Can you work these out from the model? Positions are in its coordinate system, mm. Face numbers are marked on the shaded views. Coordinates: 2 decimals unless noted, no trailing zeros. Order: outer loops, then holes, each group sorted by start corner. A loop starts at its lowest first (then second) coordinate and runs counter-clockwise, first axis right, second up. Notation, with made-up numbers: M -19,25.5 L 0,25.5 A21 ccw 0,45.5 Z; hole C 4.5,15.5 d3. An arc over 180 degrees is marked long. Answer as CSV lines item,"result". Start each with the question number.
1. If we section it at D-D (x = 0): List the corners of the cut face in (y, z) for me.
2. If we section it at A-A (y = 2): List the corners of the cut face in (x, z) for me, plus the area to 3 significant figures.
3. If we section it at C-C (z = 5): List the corners of the cut face in (x, y) for me, plus the area to 3 significant figures.
4. If we mould it in two halves opening along X, with no side actions, what happens to the marked faces 1, 2, 3 and 4? For each: released by +X, released by -X, zero draft, split by the parting line, or undercut.
5. If we section it at B-B (x = 2): List the corners of the cut face in (y, z) for me.
6. I need wall thicknesses on line 1 along Z through (x, y) = (0, 1); line 2 along X through (y, z) = (1, 3.75); line 3 along Z through (x, y) = (1, 4). Which ranges of each line are inside material? Lowest first, please. Write a range as from..to.
```python
from build123d import *

# Parameters (mm, degrees)
F0_W     = 10
F0_H     = 10
F1_DEPTH = 10
F2_R     = 2.5
F3_DEPTH = 10.1
F4_R     = 1


with BuildPart() as f1:
    # F0 (on Top) → F1 (new body)
    with BuildSketch(Plane.XY):
        Rectangle(F0_W, F0_H)
    extrude(amount=F1_DEPTH)

    # F2 (on face) → F3 (cut)
    with BuildSketch(Plane.XZ.offset(5)):
        with Locations((0, 5)):
            Circle(F2_R)
    extrude(amount=-F3_DEPTH, mode=Mode.SUBTRACT)

    # F4
    f4_edges = [f1.edges().sort_by_distance(p)[0] for p in [
        (5, 0, 10),
        (0, 5, 10),
        (-5, 0, 10),
        (0, -5, 10),
        (5, 0, 0),
        (0, 5, 0),
        (-5, 0, 0),
        (0, -5, 0),
    ]]
    fillet(f4_edges, radius=F4_R)


solid = f1.part
```
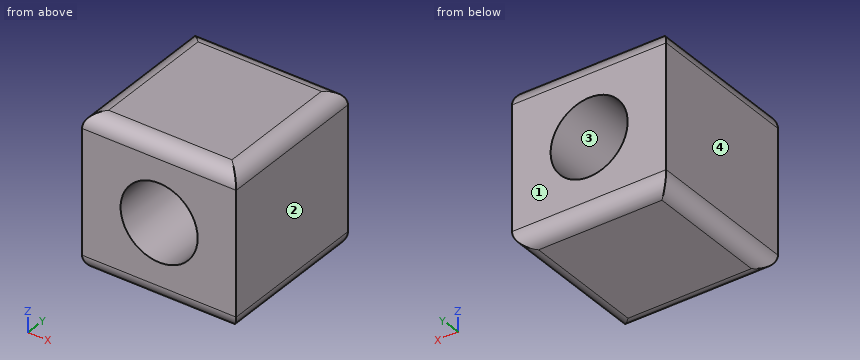
Solved:
1,outline,"M -5,1 A1 ccw -4,0 L 4,0 A1 ccw 5,1 L 5,2.5 L -5,2.5 Z; M -5,7.5 L 5,7.5 L 5,9 A1 ccw 4,10 L -4,10 A1 ccw -5,9 Z"
2,outline,"M -5,1 A1 ccw -4,0 L 4,0 A1 ccw 5,1 L 5,9 A1 ccw 4,10 L -4,10 A1 ccw -5,9 Z; hole C 0,5 d5"
2,area,"79.5 mm²"
3,outline,"M -5,-5 L -2.5,-5 L -2.5,5 L -5,5 Z; M 2.5,-5 L 5,-5 L 5,5 L 2.5,5 Z"
3,area,"50.0 mm²"
4,face 1,"zero draft"
4,face 2,"released by +X"
4,face 3,"undercut"
4,face 4,"released by -X"
5,outline,"M -5,1 A1 ccw -4,0 L 4,0 A1 ccw 5,1 L 5,3.5 L -5,3.5 Z; M -5,6.5 L 5,6.5 L 5,9 A1 ccw 4,10 L -4,10 A1 ccw -5,9 Z"
6,line 1,"0..2.5, 7.5..10"
6,line 2,"-5..-2.17, 2.17..5"
6,line 3,"0..2.71, 7.29..10"
